Verification items for the finished model (mm, model axes). Face numbers are marked on the shaded views. A direction names the side the tool comes from. Give positions to 0.01 mm unless a question says otherwise; leave off trailing zeros. Write each loop counter-clockwise with the first axis right and the second up, starting at its lowest first coordinate (ties: lowest second). Pieces come first, ordered by that corner, then holes. Notation, with made-up numbers: (35, 18.25) -> (46, 18.25) arc R21 ccw to (46, 47.25) -> close; hole circle Ø7 at (-16.75, 22.25). An arc over 180 degrees is marked (long way). Use CSV: the item, a comma, the result in double quotes. Start each with the question number.
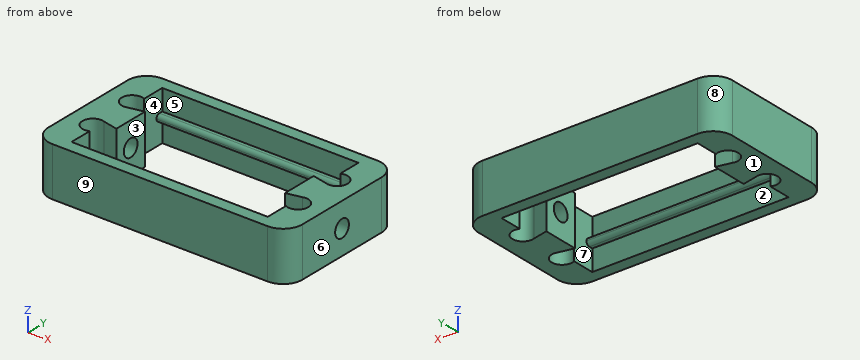
```python
from build123d import *

# Parameters (mm, degrees)
SKETCH1_W                = 26.289
SKETCH1_H                = 14.224
BOSS_EXTRUDE1_DEPTH      = 5.08
BOSS_EXTRUDE2_DEPTH      = 0.375
BOSS_EXTRUDE2_DEPTH_BACK = 0.375
SKETCH2_W                = 20.300617312
SKETCH2_H                = 0.75
FILLET1_R                = 0.375
FILLET2_R                = 2
SKETCH3_R                = 0.889
CUT_EXTRUDE1_DEPTH       = 24.13


with BuildPart() as part:
    # Sketch1 → Boss-Extrude1 (new body)
    with BuildSketch(Plane.XY):
        with Locations((13.1445, 7.112)):
            Rectangle(SKETCH1_W, SKETCH1_H)
        with BuildLine():
            ThreePointArc((2.994191344, 10.624), (1.457238853, 9.709108648), (2.886694423, 8.633977996))
            Line((2.886694423, 8.633977996), (4.417480803, 8.964165012))
            Line((4.417480803, 8.964165012), (4.417480803, 5.259834988))
            Line((4.417480803, 5.259834988), (2.886694423, 5.590022004))
            ThreePointArc((2.886694423, 5.590022004), (1.457238853, 4.514891352), (2.994191344, 3.6))
            Line((2.994191344, 3.6), (2.994191344, 1.25))
            Line((2.994191344, 1.25), (23.294808656, 1.25))
            Line((23.294808656, 1.25), (23.294808656, 3.6))
            ThreePointArc((23.294808656, 3.6), (24.831761147, 4.514891352), (23.402305577, 5.590022004))
            Line((23.402305577, 5.590022004), (21.871519197, 5.259834988))
            Line((21.871519197, 5.259834988), (21.871519197, 8.964165012))
            Line((21.871519197, 8.964165012), (23.402305577, 8.633977996))
            ThreePointArc((23.402305577, 8.633977996), (24.831761147, 9.709108648), (23.294808656, 10.624))
            Line((23.294808656, 10.624), (23.294808656, 12.974))
            Line((23.294808656, 12.974), (2.994191344, 12.974))
            Line((2.994191344, 12.974), (2.994191344, 10.624))
        make_face(mode=Mode.SUBTRACT)
    extrude(amount=BOSS_EXTRUDE1_DEPTH)

    # Sketch2 → Boss-Extrude2 (add, two sides: drawn at the far end of the back side and taken through both)
    with BuildSketch(Plane.XY.offset(2.54).offset(-BOSS_EXTRUDE2_DEPTH_BACK)):
        with Locations((13.1445, 1.625)):
            Rectangle(SKETCH2_W, SKETCH2_H)
        with Locations((13.1445, 12.599)):
            Rectangle(SKETCH2_W, SKETCH2_H)
    extrude(amount=BOSS_EXTRUDE2_DEPTH + BOSS_EXTRUDE2_DEPTH_BACK)

    # Fillet1
    fillet1_edges = [part.edges().sort_by_distance(p)[0] for p in [
        (13.1445, 12.224, 2.165),
        (13.1445, 12.224, 2.915),
        (13.1445, 2, 2.165),
        (13.1445, 2, 2.915),
    ]]
    fillet(fillet1_edges, radius=FILLET1_R - 0.0001)  # a hair under: the kernel refuses the full size

    # Fillet2
    fillet2_edges = [part.edges().sort_by_distance(p)[0] for p in [
        (0, 0, 2.54),
        (0, 14.224, 2.54),
        (26.289, 14.224, 2.54),
        (26.289, 0, 2.54),
    ]]
    fillet(fillet2_edges, radius=FILLET2_R)

    # Sketch3 → Cut-Extrude1 (cut)
    with BuildSketch(Plane(origin=(26.289, 0, 0), x_dir=(0, 0, -1), z_dir=(1, 0, 0))):
        with Locations((-2.54, 7.112)):
            Circle(SKETCH3_R)
    extrude(amount=-CUT_EXTRUDE1_DEPTH, mode=Mode.SUBTRACT)


solid = part.part
```
(1) Section check D-D on z = 0.75. Record the cut outline in (x, y).
(2) Set-up check for the marked faces 1, 2, 3, 4 and 5: record each of +Z, -Z, +X, -X, +Y, -Y from which the full face is reachable in a straight line by a thin tool's end or side.
(3) Thickness scan on line 1 (Y direction, x = 2.6, z = 2.54); line 2 (X direction, y = 2.75, z = 0.6); line 3 (X direction, y = 8, z = 3.2). Record the ranges inside material, lowest first. Write a range as from..to.
(4) Section check B-B on y = 11.25. Record the cut outline in (x, z).
(5) Go/stop test with flat-tipped pins: pin 1 (1 mm diameter, centred on x = 11.5, y = 3, fed in from +Z); pin 2 (1.1 mm diameter, centred on y = 7.112, z = 2.54, fed in from +X). Record where each tip stops, or that it passes through.
(6) Section check A-A on x = 2.5. Record the cut outline in (y, z), then the cut area to 3 significant figures.
(7) Draft check along X on the marked faces 6, 7, 8 and 9. Enter one of: released by +X, released by -X, zero draft, split by the parting line, or undercut.
Data:
1,outline,"(0, 2) arc R2 ccw to (2, 0) -> (24.29, 0) arc R2 ccw to (26.29, 2) -> (26.29, 12.22) arc R2 ccw to (24.29, 14.22) -> (2, 14.22) arc R2 ccw to (0, 12.22) -> close; hole (2.89, 5.59) arc R1.08 ccw (long way) to (2.99, 3.6) -> (2.99, 1.25) -> (23.29, 1.25) -> (23.29, 3.6) arc R1.08 ccw (long way) to (23.4, 5.59) -> (21.87, 5.26) -> (21.87, 8.96) -> (23.4, 8.63) arc R1.08 ccw (long way) to (23.29, 10.62) -> (23.29, 12.97) -> (2.99, 12.97) -> (2.99, 10.62) arc R1.08 ccw (long way) to (2.89, 8.63) -> (4.42, 8.96) -> (4.42, 5.26) -> close"
2,face 1,"-Z, +X, -X, +Y, -Y"
2,face 2,"-Z"
2,face 3,"+Z, -Z"
2,face 4,"none"
2,face 5,"+Z"
3,line 1,"y = 0..3.5, 5.65..6.22, 8..8.58, 10.73..14.22"
3,line 2,"x = 0..2.99, 23.29..26.29"
3,line 3,"x = 0..4.42, 21.87..26.29"
4,outline,"(0, 0) -> (2.99, 0) -> (2.99, 5.08) -> (0, 5.08) -> close; (23.29, 0) -> (26.29, 0) -> (26.29, 5.08) -> (23.29, 5.08) -> close"
5,pin 1,"passes through"
5,pin 2,"stops at x = 2.16"
6,outline,"(0, 0) -> (3.5, 0) -> (3.5, 5.08) -> (0, 5.08) -> close; (5.65, 0) -> (8.57, 0) -> (8.57, 5.08) -> (5.65, 5.08) -> close; (10.73, 0) -> (14.22, 0) -> (14.22, 5.08) -> (10.73, 5.08) -> close; hole circle Ø1.78 at (7.11, 2.54)"
6,area,"47.9 mm2"
7,face 6,"released by +X"
7,face 7,"undercut"
7,face 8,"released by -X"
7,face 9,"zero draft"
